```python
from build123d import *

# Parameters (mm, degrees)
SKETCH_1_W          = 45
SKETCH_1_H          = 8
EXTRUDE_1_DEPTH     = 9
CUT_EXTRUDE_1_DEPTH = 26.51960031
SKETCH_4_W          = 6.6
SKETCH_4_H          = 2.5
CUT_EXTRUDE_2_DEPTH = 47.583258795
CUT_EXTRUDE_3_DEPTH = 30.904013109
FILLET_1_R          = 1
SCALE_1_SCALE       = 2.666666667


with BuildPart() as part:
    # 草图1 → 凸台-拉伸1 (new, symmetric)
    with BuildSketch(Plane.XY):
        with Locations((0, 4)):
            Rectangle(SKETCH_1_W, SKETCH_1_H)
    extrude(amount=EXTRUDE_1_DEPTH, both=True)

    # 草图2 → 切除-拉伸1 (cut, through all)
    with BuildSketch(Plane(origin=(0, 8, 0), x_dir=(1, 0, 0), z_dir=(0, 1, 0))):
        with BuildLine():
            Line((-14.5, 3.3), (-3.5, 3.3))
            ThreePointArc((-3.5, 3.3), (-0.2, 0), (-3.5, -3.3))
            Line((-3.5, -3.3), (-14.5, -3.3))
            ThreePointArc((-14.5, -3.3), (-17.8, 0), (-14.5, 3.3))
        make_face()
    extrude(amount=-CUT_EXTRUDE_1_DEPTH, mode=Mode.SUBTRACT)

    # 草图4 → 切除-拉伸2 (cut, through all)
    with BuildSketch(Plane(origin=(22.5, 0, 0), x_dir=(0, 0, -1), z_dir=(1, 0, 0))):
        with Locations((0, 1.25)):
            Rectangle(SKETCH_4_W, SKETCH_4_H)
    extrude(amount=-CUT_EXTRUDE_2_DEPTH, mode=Mode.SUBTRACT)

    # 草图5 → 切除-拉伸3 (cut, through all)
    with BuildSketch(Plane.XY.offset(9)):
        Polygon((-17.5, 1), (-11.5, 1), (-9.767949192, 0), (-19.232050808, 0), align=None)
    extrude(amount=-CUT_EXTRUDE_3_DEPTH, mode=Mode.SUBTRACT)

    # 圆角1
    fillet_1_edges = [part.edges().sort_by_distance(p)[0] for p in [
        (22.5, 0, -6.15),
        (-22.5, 0, -6.15),
        (-22.5, 8, 0),
        (22.5, 8, 0),
        (22.5, 0, 6.15),
        (-22.5, 0, 6.15),
    ]]
    fillet(fillet_1_edges, radius=FILLET_1_R)


with BuildPart() as part_1:
    # 缩放比例1: scaled about (1.300247122, 4.318589473, 0)
    add(part.part.scale(SCALE_1_SCALE).moved(Location((-2.167078537, -7.197649122, 0))))


solid = part_1.part
```
Geometry: final body of the model. Coordinates: model frame, mm. A direction names the side the tool comes from. Coordinates: 2 decimals unless noted, no trailing zeros. Order: outer loops, then holes, each group sorted by start corner. A loop starts at its lowest first (then second) coordinate and runs counter-clockwise, first axis right, second up. Notation, with made-up numbers: (15, -22) - (61, -22) arc R3 ccw to (61, -17) - close; hole circle Ø7 at (55, 68). An arc over 180 degrees is marked (long way). Write each question's results on one line, items separated by ' | '.
1) Pull-direction query (Z, two-part tool) for faces 1 (the cylindrical face through (-2.703, 6.905, -0.194)), 2 (the flat face through (24, -0.531, 0)), 3 (the flat face through (-30.557, -5.846, 16.506)), 4 (the flat face through (-3, 4, 24)); classes: pulls with the +Z half, pulls with the -Z half, needs draft (parallel to the pull), parting line crosses it, or undercut.
Results list:
face 1: undercut | face 2: undercut | face 3: needs draft | face 4: pulls with the +Z half
2) Line query: line 1 (Z direction, x = -22.5, y = 3.75); line 2 (X direction, y = 2, z = -0.5); line 3 (Y direction, x = 2, z = -1.5). Output: solid intervals per line, ascending. Write a range as from..to.
Results list:
line 1: -24..-8.8, 8.8..24 | line 2: -62.17..-49.62, -2.71..57.83 | line 3: -0.53..14.14
3) Pin query (flat end, axial travel): pin 1 (5.5 mm diameter, centred on x = 30.5, z = -2.5, fed in from -Y); pin 2 (5 mm diameter, centred on x = -18.5, z = -6, fed in from +Y); pin 3 (4.5 mm diameter, centred on x = -40.5, z = 15.5, fed in from -Y). Return the tip coordinate at first contact, or that it passes through.
Results list:
pin 1: y = -0.53 | pin 2: through | pin 3: y = -4.53
4) Section A-A, the plane z = 0. Return loops of the section in (x, y).
Results list:
outline: (-62.17, -0.53) - (-49.63, -0.53) - (-49.63, 14.14) - (-59.5, 14.14) arc R2.67 ccw to (-62.17, 11.47) - close; (-2.7, -0.53) - (57.83, -0.53) - (57.83, 11.47) arc R2.67 ccw to (55.17, 14.14) - (-2.7, 14.14) - close
5) Section B-B, the plane y = 2. Return loops of the section in (x, z), plus the area to 3 significant figures.
Results list:
outline: (-62.17, -24) - (57.83, -24) - (57.83, 24) - (-62.17, 24) - close; hole (-40.83, -8.8) - (-11.5, -8.8) arc R8.8 ccw to (-11.5, 8.8) - (-40.83, 8.8) arc R8.8 ccw to start | area: 5,000 mm^2
6) Set-up query: faces 5 (the flat face through (-1, -1, -8.8)), 6 (the flat face through (57.833, 3, 0)), 7 (the flat face through (-41, -4.531, -16)), 8 (the cylindrical face through (-49.63, 6.91, 0.19)). Return all of +Z, -Z, +X, -X, +Y, -Y with unobstructed straight access to the full face (end or side cutting, diameter ignored); none if empty.
Results list:
face 5: -Y | face 6: +Z, -Z, +X, +Y, -Y | face 7: +Z, -Z, -Y | face 8: +Y, -Y
7) Section C-C, the plane x = 44. Return loops of the section in (y, z), plus the area to 3 significant figures.
Results list:
outline: (-7.2, -24) - (14.14, -24) - (14.14, 24) - (-7.2, 24) - (-7.2, 8.8) - (-0.53, 8.8) - (-0.53, -8.8) - (-7.2, -8.8) - close | area: 907 mm^2
8) Section D-D, the plane z = 17.5. Return loops of the section in (x, y), plus the area to 3 significant figures.
Results list:
outline: (-62.17, -4.53) arc R2.67 ccw to (-59.5, -7.2) - (-53.45, -7.2) - (-48.83, -4.53) - (-32.83, -4.53) - (-28.21, -7.2) - (55.17, -7.2) arc R2.67 ccw to (57.83, -4.53) - (57.83, 11.47) arc R2.67 ccw to (55.17, 14.14) - (-59.5, 14.14) arc R2.67 ccw to (-62.17, 11.47) - close | area: 2,500 mm^2
